Read the model definition and answer for the solid it produces. Units are mm, in the model's axes. Face numbers are marked on the shaded views. A direction names the side the tool comes from. Round coordinates to 2 decimals unless told otherwise and drop trailing zeros. Order: outer loops, then holes, each group sorted by start corner. A loop starts at its lowest first (then second) coordinate and runs counter-clockwise, first axis right, second up. Notation, with made-up numbers: (-23, 34.5) -> (26, 34.5) arc R17 ccw to (26, 55.5) -> close; hole circle Ø8 at (43.5, 26). An arc over 180 degrees is marked (long way). One line per item, written item: value. Start each with the question number.
1. Section C-C (z = 4.5) is taken. Give the vertices of the cut face in (x, y).
2. Flat-ended cylindrical pins translate along their axes: pin 1 Ø3 at (x, y) = (0, -2) entering from +Z; pin 2 Ø6 at (x, y) = (-13, -5.5) entering from -Z. Find the tip coordinate at first contact, or state that the pin passes through.
3. Section B-B (x = -1) is taken. Give the vertices of the cut face in (y, z).
4. Consider line 1 (X direction, y = -1.5, z = 7.5); line 2 (Y direction, x = 0, z = 1.45); line 3 (X direction, y = -1.75, z = 2.5). Determine where each line is inside the solid, lowest interval first.
5. Section A-A (y = -2) is taken. Give the vertices of the cut face in (x, z), then the cut area to 3 significant figures.
6. Section D-D (z = 1.5) is taken. Give the vertices of the cut face in (x, y), then the cut area to 3 significant figures.
7. The mould has two halves that part along X. Classify the marked faces 3, 4, 5 and 6: released by +X, released by -X, zero draft, split by the parting line, or undercut.
8. For the marked faces 1 and 2, determine the directions among +Z, -Z, +X, -X, +Y, -Y from which every point of the face is accessible in a straight line to the end or side of a thin tool.
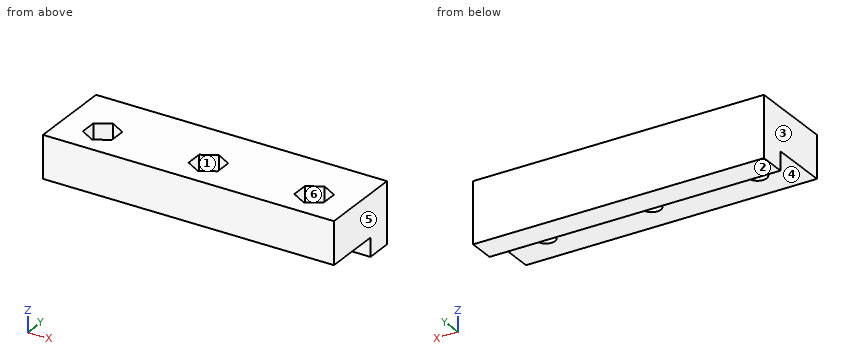
from build123d import *

# Parameters (mm, degrees)
F0_W     = 55
F0_H     = 5
F0_H_2   = 11
F1_DEPTH = 8
F0_R     = 1.75
F2_DEPTH = 4
F3_DEPTH = 3.5


with BuildPart() as f1:
    # F0 (on Top) → F1 (new body)
    with BuildSketch(Plane.XY):
        with Locations((0, 5.5)):
            Rectangle(F0_W, F0_H)
        with Locations((0, -2.5)):
            Rectangle(F0_W, F0_H_2)
        Polygon((-20, -5.175426), (-22.75, -3.587713), (-22.75, -0.412287), (-20, 1.175426), (-17.25, -0.412287), (-17.25, -3.587713), align=None, mode=Mode.SUBTRACT)
        Polygon((0, -5.175426), (-2.75, -3.587713), (-2.75, -0.412287), (0, 1.175426), (2.75, -0.412287), (2.75, -3.587713), align=None, mode=Mode.SUBTRACT)
        Polygon((20, 1.175426), (22.75, -0.412287), (22.75, -3.587713), (20, -5.175426), (17.25, -3.587713), (17.25, -0.412287), align=None, mode=Mode.SUBTRACT)
    extrude(amount=F1_DEPTH)

    # F0 (on Top) → F2 (join)
    with BuildSketch(Plane.XY):
        Polygon((-22.75, -0.412287), (-22.75, -3.587713), (-20, -5.175426), (-17.25, -3.587713), (-17.25, -0.412287), (-20, 1.175426), align=None)
        with Locations((-20, -2)):
            Circle(F0_R, mode=Mode.SUBTRACT)
        Polygon((-2.75, -0.412287), (-2.75, -3.587713), (0, -5.175426), (2.75, -3.587713), (2.75, -0.412287), (0, 1.175426), align=None)
        with Locations((0, -2)):
            Circle(F0_R, mode=Mode.SUBTRACT)
        Polygon((22.75, -3.587713), (22.75, -0.412287), (20, 1.175426), (17.25, -0.412287), (17.25, -3.587713), (20, -5.175426), align=None)
        with Locations((20, -2)):
            Circle(F0_R, mode=Mode.SUBTRACT)
    extrude(amount=F2_DEPTH)

    # F0 (on Top) → F3 (join)
    with BuildSketch(Plane.XY):
        with Locations((0, 5.5)):
            Rectangle(F0_W, F0_H)
    extrude(amount=-F3_DEPTH)


solid = f1.part
Answer:
1. outline: (-27.5, -8) -> (27.5, -8) -> (27.5, 8) -> (-27.5, 8) -> close; hole (-22.75, -3.59) -> (-20, -5.18) -> (-17.25, -3.59) -> (-17.25, -0.41) -> (-20, 1.18) -> (-22.75, -0.41) -> close; hole (-2.75, -3.59) -> (0, -5.18) -> (2.75, -3.59) -> (2.75, -0.41) -> (0, 1.18) -> (-2.75, -0.41) -> close; hole (17.25, -3.59) -> (20, -5.18) -> (22.75, -3.59) -> (22.75, -0.41) -> (20, 1.18) -> (17.25, -0.41) -> close
2. pin 1: through
2. pin 2: z = 0
3. outline: (-8, 0) -> (-3.44, 0) -> (-3.44, 4) -> (-4.6, 4) -> (-4.6, 8) -> (-8, 8) -> close; (-0.56, 0) -> (3, 0) -> (3, -3.5) -> (8, -3.5) -> (8, 8) -> (0.6, 8) -> (0.6, 4) -> (-0.56, 4) -> close
4. line 1: -27.5 to -22.75, -17.25 to -2.75, 2.75 to 17.25, 22.75 to 27.5
4. line 2: -8 to -3.75, -0.25 to 8
4. line 3: -27.5 to -21.73, -18.27 to -1.73, 1.73 to 18.27, 21.73 to 27.5
5. outline: (-27.5, 0) -> (-21.75, 0) -> (-21.75, 4) -> (-22.75, 4) -> (-22.75, 8) -> (-27.5, 8) -> close; (-18.25, 0) -> (-1.75, 0) -> (-1.75, 4) -> (-2.75, 4) -> (-2.75, 8) -> (-17.25, 8) -> (-17.25, 4) -> (-18.25, 4) -> close; (1.75, 0) -> (18.25, 0) -> (18.25, 4) -> (17.25, 4) -> (17.25, 8) -> (2.75, 8) -> (2.75, 4) -> (1.75, 4) -> close; (21.75, 0) -> (27.5, 0) -> (27.5, 8) -> (22.75, 8) -> (22.75, 4) -> (21.75, 4) -> close
5. area: 332 mm^2
6. outline: (-27.5, -8) -> (27.5, -8) -> (27.5, 8) -> (-27.5, 8) -> close; hole circle Ø3.5 at (-20, -2); hole circle Ø3.5 at (0, -2); hole circle Ø3.5 at (20, -2)
6. area: 851 mm^2
7. face 3: released by -X
7. face 4: zero draft
7. face 5: released by +X
7. face 6: undercut
8. face 1: +Z
8. face 2: -Z, +X, -X, +Y, -Y
